Input: part model. Units: mm. Frame: model coordinates. A direction names the side the tool comes from. Coordinates: 2 decimals unless noted, no trailing zeros. Loops run counter-clockwise (first coordinate to the right, second up) from the corner with the lowest first, then second, coordinate; pieces in that order, holes last. Notation, with made-up numbers: (50.5, 55.25) -> (88.5, 55.25) arc R10 cw to (88.5, 59.25) -> close; hole circle Ø9 at (16.25, 6.5). An arc over 180 degrees is marked (long way). Put each result on its own line as item: value. Start each with the question number.
1) Material intervals for L1, parallel to Z at x = -65.5, y = 4.5; L2, parallel to Z at x = -15, y = 7.25; L3, parallel to X at y = 6.75, z = -65, sorted ascending.
2) Cut plane A-A (x = -15). Return the cut outline in (y, z), plus the area to 3 significant figures.
3) Set-up query: faces 1 (the flat face through (0, 5, -35)), 2 (the flat face through (-66, 3, -53)). Return all of +Z, -Z, +X, -X, +Y, -Y with unobstructed straight access to the full face (end or side cutting, diameter ignored); none if empty.
4) Contact query for flat-ended pins moving along their axis: P1, Ø0.9, axis at x = -66, z = -54, coming from the +Y side; P2, Ø2.5, axis at x = -85, z = -65, coming from the +Y side. Output: stop coordinate, or through.
5) Pull-direction query (X, two-part tool) for faces 3 (the cylindrical face through (-2, 5.1, -67.9)), 4 (the flat face through (-85, 2, -65)), 5 (the flat face through (-46, 10, -35)); classes: pulls with the +X half, pulls with the -X half, needs draft (parallel to the pull), parting line crosses it, or undercut.
6) Cut plane C-C (z = -25.25). Return the cut outline in (x, y).
7) Cut plane D-D (x = -65.5). Return the cut outline in (y, z).
8) Cut plane B-B (y = 9). Return the cut outline in (x, z), plus the area to 3 significant figures.
Autodesk Inventor part; units mm, degrees
ref_plane "YZ Plane" through (0, 0, 0) normal (1, 0, 0) x (0, 1, 0)
ref_plane "XZ Plane" through (0, 0, 0) normal (0, 1, 0) x (-1, 0, 0)
ref_plane "XY Plane" through (0, 0, 0) normal (0, 0, 1) x (1, 0, 0)
sketch "Sketch1" plane through (0, 0, 0) normal (0, 1, 0) x (-1, 0, 0)
  line L0 (0, 0) -> (0, -70)
  line L1 (0, -70) -> (90, -70)
  line L2 (90, -70) -> (90, 0)
  line L3 (90, 0) -> (0, 0)
  circle A0 centre (85, -65) radius 1.6095
  circle A1 centre (85, -5) radius 1.6095
  circle A2 centre (85, -5) radius 1.6095
  circle A3 centre (85, -65) radius 1.6095
  circle A4 centre (5, -65) radius 1.6095
  circle A5 centre (5, -5) radius 1.6095
  circle A6 centre (5, -65) radius 1.6095
  circle A7 centre (5, -5) radius 1.6095
  dimension "d0" = 70
  dimension "d1" = 90
  dimension "d5" = 5
  dimension "d6" = 3.2191
extrude "Extrusion1" add sketch "Sketch1" along normal blind 15
sketch "Sketch2" plane through (0, 15, 0) normal (0, 1, 0) x (1, 0, 0)
  line L0 (-90, 70) -> (-90, 0)
  line L1 (-90, 0) -> (0, 0)
  line L2 (-90, 0) -> (0, 0)
  line L3 (0, 70) -> (-90, 70)
  line L4 (0, 0) -> (0, 70)
  line L5 (0, 70) -> (-90, 70)
  line L6 (-90, 70) -> (-90, 0)
extrude "Extrusion2" cut sketch "Sketch2" against normal blind 5
fillet "Fillet1" radius 7 4 edges at (-90, 5, -70) (-90, 5, 0) (0, 5, -70) (0, 5, 0)
sketch "Sketch3" plane through (0, 0, 0) normal (0, -1, 0) x (1, 0, 0)
  circle A0 centre (-85, -65) radius 1.6095
  circle A1 centre (-85, -65) radius 1.6095
  circle A2 centre (-85, -5) radius 1.6095
  circle A3 centre (-85, -5) radius 1.6095
  circle A4 centre (-5, -5) radius 1.6095
  circle A5 centre (-5, -5) radius 1.6095
  circle A6 centre (-5, -65) radius 1.6095
  circle A7 centre (-5, -65) radius 1.6095
  point P0 (0, 0)
extrude "Extrusion3" add sketch "Sketch3" against normal blind 2
sketch "Sketch4" plane through (0, 10, 0) normal (0, 1, 0) x (1, 0, 0)
  point P0 (0, 0)
sketch "Sketch5" plane through (0, 10, 0) normal (0, 1, 0) x (1, 0, 0)
  circle A0 centre (-15, 12.25) radius 1.5
  circle A1 centre (-65.5, 53.25) radius 1.5
  circle A2 centre (-65.5, 25.25) radius 1.5
  point P0 (0, 0)
extrude "Extrusion4" cut sketch "Sketch5" against normal blind 7
properties part number "Módulo de fixação Arduíno" material "PPS Plastic"
Results found:
1. L1: z = -70 to -54.75, -51.75 to -26.75, -23.75 to 0
1. L2: z = -70 to -13.75, -10.75 to 0
1. L3: x = -89.71 to -86.61, -83.39 to -6.61, -3.39 to -0.29
2. outline: (0, -70) -> (10, -70) -> (10, -13.75) -> (3, -13.75) -> (3, -10.75) -> (10, -10.75) -> (10, 0) -> (0, 0) -> close
2. area: 679 mm2
3. face 1: +Z, -Z, +X, +Y, -Y
3. face 2: +Y
4. P1: stops at y = 3
4. P2: stops at y = 2
5. face 3: pulls with the +X half
5. face 4: undercut
5. face 5: needs draft
6. outline: (-90, 0) -> (0, 0) -> (0, 10) -> (-64, 10) -> (-64, 3) -> (-67, 3) -> (-67, 10) -> (-90, 10) -> close
7. outline: (0, -70) -> (10, -70) -> (10, -54.75) -> (3, -54.75) -> (3, -51.75) -> (10, -51.75) -> (10, -26.75) -> (3, -26.75) -> (3, -23.75) -> (10, -23.75) -> (10, 0) -> (0, 0) -> close
8. outline: (-90, -63) arc R7 ccw to (-83, -70) -> (-7, -70) arc R7 ccw to (0, -63) -> (0, -7) arc R7 ccw to (-7, 0) -> (-83, 0) arc R7 ccw to (-90, -7) -> close; hole circle Ø3.22 at (-85, -65); hole circle Ø3.22 at (-85, -5); hole circle Ø3 at (-65.5, -53.25); hole circle Ø3 at (-65.5, -25.25); hole circle Ø3 at (-15, -12.25); hole circle Ø3.22 at (-5, -65); hole circle Ø3.22 at (-5, -5)
8. area: 6,200 mm2
